Could you check a few things on this model? Use its own coordinates, in mm. A direction names the side the tool comes from. Give positions to 0.01 mm unless a question says otherwise; leave off trailing zeros. Order: outer loops, then holes, each group sorted by start corner. A loop starts at its lowest first (then second) coordinate and runs counter-clockwise, first axis right, second up. Notation, with made-up numbers: (-34, 74) -> (21, 74) arc R37 ccw to (21, 111) -> close; hole circle Ø8 at (-21, 8). An arc over 180 degrees is marked (long way). Answer as CSV lines item,"result". Start each with the question number.
(1) I want a section at A-A (z = -0.5). Please give me the cut outline in (x, y), plus the area to 3 significant figures.
(2) I need wall thicknesses on L1, parallel to X at y = -0.25, z = -1.3. Which ranges of the line are inside material? Lowest first, please.
(3) We'd pull the mould along Y, two halves only. Please class faces 4 (the face through (27, -11, 0)), 5 (the face through (2, 5, 0)), 6 (the face through (54, -8, 0)), 7 (the face through (2, -5, 0)): released by +Y, released by -Y, zero draft, split by the parting line, or undercut.
(4) Will this pin go through, and if not, where does the flat tip stop? pin 1 Ø0.9 at (y, z) = (2, 0) entering from +X.
(5) I want a section at B-B (y = -4.5). Please give me the cut outline in (x, z).
(6) On a 3-axis mill with a long thin cutter (end or side, diameter ignored), from which of +Z, -Z, +X, -X, +Y, -Y can I reach the whole of each face in a straight line? I mean faces 1 (the face through (51, 0, 0)), 2 (the face through (27, 0, 1.5)), 3 (the face through (4, 0, 0)). Say none if no direction works.
```python
from build123d import *

# Parameters (mm, degrees)
BOSS_EXTRUDE1_DEPTH = 1.5
SKETCH2_W           = 3
SKETCH2_H           = 10
CUT_EXTRUDE1_DEPTH  = 56.865910894
SKETCH3_W           = 55
SKETCH3_H           = 25
CUT_EXTRUDE2_DEPTH  = 56.865910894
SKETCH6_W           = 15
SKETCH6_H           = 3
CUT_EXTRUDE5_DEPTH  = 56.865910894


with BuildPart() as part:
    # Sketch1 → Boss-Extrude1 (new, symmetric)
    with BuildSketch(Plane.XY):
        Polygon((-20, -11), (20, -11), (20, -14), (35, -14), (35, -11), (54, -11), (54, 11), (-54, 11), (-54, -11), (-35, -11), (-35, -14), (-20, -14), align=None)
    extrude(amount=BOSS_EXTRUDE1_DEPTH, both=True)

    # Sketch2 → Cut-Extrude1 (cut, through all)
    with BuildSketch(Plane.XY.offset(1.5)):
        with Locations((2.5, 0)):
            Rectangle(SKETCH2_W, SKETCH2_H)
        with Locations((52.5, 0)):
            Rectangle(SKETCH2_W, SKETCH2_H)
    extrude(amount=-CUT_EXTRUDE1_DEPTH, mode=Mode.SUBTRACT)

    # Sketch3 → Cut-Extrude2 (cut, through all)
    with BuildSketch(Plane.XY.offset(1.5)):
        with Locations((-26.5, -1.5)):
            Rectangle(SKETCH3_W, SKETCH3_H)
    extrude(amount=-CUT_EXTRUDE2_DEPTH, mode=Mode.SUBTRACT)

    # Sketch6 → Cut-Extrude5 (cut, through all)
    with BuildSketch(Plane.XY.offset(1.5)):
        with Locations((27.5, -12.5)):
            Rectangle(SKETCH6_W, SKETCH6_H)
    extrude(amount=-CUT_EXTRUDE5_DEPTH, mode=Mode.SUBTRACT)


solid = part.part
```
Final values:
1,outline,"(1, -11) -> (54, -11) -> (54, -5) -> (51, -5) -> (51, 5) -> (54, 5) -> (54, 11) -> (1, 11) -> (1, 5) -> (4, 5) -> (4, -5) -> (1, -5) -> close"
1,area,"1,110 mm²"
2,L1,"4 to 51"
3,face 4,"released by -Y"
3,face 5,"undercut"
3,face 6,"zero draft"
3,face 7,"undercut"
4,pin 1,"x = 51"
5,outline,"(4, -1.5) -> (51, -1.5) -> (51, 1.5) -> (4, 1.5) -> close"
6,face 1,"+Z, -Z, +X"
6,face 2,"+Z, +X, -X, +Y, -Y"
6,face 3,"+Z, -Z, -X"
